Build history of the part. All positions in model axes, mm. A direction names the side the tool comes from. Give positions to 0.01 mm unless a question says otherwise; leave off trailing zeros. Write each loop counter-clockwise with the first axis right and the second up, starting at its lowest first coordinate (ties: lowest second). Pieces come first, ordered by that corner, then holes. Notation, with made-up numbers: (-28, -27) -> (28, -27) arc R19 cw to (28, -20) -> close; hole circle Ø5 at (43.5, 44.25). An arc over 180 degrees is marked (long way). Put each result on its own line as item: value. Start each with the question number.
Item 1: Flat gauge pins, fed straight in: pin 1 Ø5.5 at (x, y) = (-19.02, 6.18) entering from +Z; pin 2 Ø1.5 at (y, z) = (6.5, 0.5) entering from -X; pin 3 Ø5 at (y, z) = (-21, 4.5) entering from +X. Where does each tip first touch, or does it go through?
Item 2: Slice it at C-C, the plane z = 4.25. List the corners of the cut face in (x, y), plus the area to 3 significant figures.
Item 3: Tool access for faces 5 (the flat face through (0, -16, 6)), 6 (the flat face through (-12, -13.8, -1.8)), 7 (the cylindrical face through (-15.683, 7.232, 4.718)): list every direction of +Z, -Z, +X, -X, +Y, -Y with a clear straight run to the whole face (end or side of a thin tool).
Item 4: Drill centre lines: line 1 along X through (y, z) = (7.5, 3); line 2 along X through (y, z) = (7, 4); line 3 along Y through (x, z) = (10.5, 4.5). Where is each one in solid material? Low to high.
Item 5: Two-plate mould, pull along Y, no slides. Class faces 1 (the flat face through (-18, 4, 3.4)), 2 (the flat face through (-17, -19, 0)), 3 (the cylindrical face through (-0.46, 23.47, 4.72)), 4 (the cylindrical face through (25.865, -10.724, -2.465)): pulls with the +Y half, pulls with the -Y half, needs draft (parallel to the pull), parting line crosses it, or undercut.
Item 6: Slice it at D-D, the plane z = 1. List the corners of the cut face in (x, y), plus the area to 3 significant figures.
Item 7: Slice it at B-B, the plane z = -4. Give the number of separate pieces and of enclosed holes in the cut face, plus the area to 3 significant figures.
Item 8: Slice it at A-A, the plane y = 0. List the corners of the cut face in (x, z), plus the area to 3 significant figures.
Autodesk Inventor part; units mm, degrees
ref_plane "YZ Plane" through (0, 0, 0) normal (1, 0, 0) x (0, 1, 0)
ref_plane "XZ Plane" through (0, 0, 0) normal (0, 1, 0) x (-1, 0, 0)
ref_plane "XY Plane" through (0, 0, 0) normal (0, 0, 1) x (1, 0, 0)
sketch "스케치1" plane through (0, 0, 0) normal (0, 0, 1) x (1, 0, 0)
  circle A0 centre (0, 0) radius 24.95
  circle A1 centre (0, 0) radius 28
  circle A2 centre (0, 0) radius 15
  dimension "d0" = 49.9
  dimension "d1" = 56
  dimension "d2" = 30
extrude "돌출1" add sketch "스케치1" along normal blind 6 contours A0
extrude "돌출2" add sketch "스케치1" against normal blind 5 contours A0 | A1
sketch "스케치3" plane through (0, 0, 6) normal (0, 0, 1) x (1, 0, 0)
  circle A0 centre (0, 0) radius 20 construction
  circle A1 centre (0, 20) radius 2.2
  circle A2 centre (-19.0211, 6.1803) radius 2.2
  circle A3 centre (-11.7557, -16.1803) radius 2.2
  circle A4 centre (11.7557, -16.1803) radius 2.2
  circle A5 centre (19.0211, 6.1803) radius 2.2
  dimension "d9" = 40
  dimension "d10" = 4.4
  dimension "d13" = 360
extrude "돌출3" cut sketch "스케치3" against normal blind 44.5
sketch "스케치4" plane through (0, 0, -5) normal (0, 0, -1) x (-1, 0, 0)
  circle A0 centre (0, 20) radius 2.2
  line L0 (0, 15.8431) -> (-3.6, 17.9215)
  line L1 (-3.6, 17.9215) -> (-3.6, 22.0785)
  line L2 (-3.6, 22.0785) -> (0, 24.1569)
  line L3 (0, 24.1569) -> (3.6, 22.0785)
  line L4 (3.6, 22.0785) -> (3.6, 17.9215)
  line L5 (3.6, 17.9215) -> (0, 15.8431)
  point P0 (0, 0)
  dimension "d19" = 7.2
extrude "돌출4" cut sketch "스케치4" against normal blind 3.2 contours A0 | L0 L1 L2 L3 L4 L5
pattern_circular "원형 패턴1" count 5 over 360 about axis through (0, 0, 0) along (0, 0, 1) of "돌출4"
sketch "스케치6" plane through (0, 0, 6) normal (0, 0, 1) x (1, 0, 0)
  circle A0 centre (0, 20) radius 2.2
  circle A1 centre (0, 20) radius 3.5
  circle A2 centre (-19.0211, 6.1803) radius 3.5
  circle A3 centre (-11.7557, -16.1803) radius 3.5
  circle A4 centre (11.7557, -16.1803) radius 3.5
  circle A5 centre (19.0211, 6.1803) radius 3.5
  point P0 (0, 0)
  dimension "d26" = 7
  dimension "d29" = 360
extrude "돌출5" cut sketch "스케치6" against normal blind 2.6 contours A0 | A1 | A2 | A3 | A4 | A5
chamfer "모따기2" distance 1 angle 45 1 edges at (-24.95, 0, 6)
properties part number "사이클로이드 기어 축 연결 하우징"
Values follow:
1. pin 1: z = 3.4
1. pin 2: x = -27.36
1. pin 3: x = 16.74
2. outline: circle Ø49.9 at (0, 0); hole circle Ø7 at (-19.02, 6.18); hole circle Ø7 at (-11.76, -16.18); hole circle Ø30 at (0, 0); hole circle Ø7 at (0, 20); hole circle Ø7 at (11.76, -16.18); hole circle Ø7 at (19.02, 6.18)
2. area: 1,060 mm2
3. face 5: +Z, +X, -X, +Y, -Y
3. face 6: -Z
3. face 7: +Z
4. line 1: -23.8 to -20.78, -17.26 to -12.99, 12.99 to 17.26, 20.78 to 23.8
4. line 2: -23.95 to -22.42, -15.62 to -13.27, 13.27 to 15.62, 22.42 to 23.95
4. line 3: -22.63 to -19.45, -12.91 to -10.71, 10.71 to 22.63
5. face 1: undercut
5. face 2: needs draft
5. face 3: undercut
5. face 4: parting line crosses it
6. outline: circle Ø49.9 at (0, 0); hole circle Ø4.4 at (-19.02, 6.18); hole circle Ø30 at (0, 0); hole circle Ø4.4 at (-11.76, -16.18); hole circle Ø4.4 at (0, 20); hole circle Ø4.4 at (11.76, -16.18); hole circle Ø4.4 at (19.02, 6.18)
6. area: 1,170 mm2
7. separate pieces: 1
7. enclosed holes: 6
7. area: 1,530 mm2
8. outline: (-28, -5) -> (-15, -5) -> (-15, 6) -> (-23.95, 6) -> (-24.95, 5) -> (-24.95, 0) -> (-28, 0) -> close; (15, -5) -> (28, -5) -> (28, 0) -> (24.95, 0) -> (24.95, 5) -> (23.95, 6) -> (15, 6) -> close
8. area: 248 mm2
